Autodesk Inventor part; units mm, degrees
ref_plane "YZ Plane" through (0, 0, 0) normal (1, 0, 0) x (0, 1, 0)
ref_plane "XZ Plane" through (0, 0, 0) normal (0, 1, 0) x (-1, 0, 0)
ref_plane "XY Plane" through (0, 0, 0) normal (0, 0, 1) x (1, 0, 0)
sketch "Sketch1" plane through (0, 0, 0) normal (0, 1, 0) x (-1, 0, 0)
  line L0 (0, 0) -> (-76.5, 0)
  line L1 (-76.5, 0) -> (-76.5, 56.5)
  line L2 (-76.5, 56.5) -> (0, 56.5)
  line L3 (0, 56.5) -> (0, 0)
  dimension "d0" = 76.5
  dimension "d1" = 56.5
extrude "Extrusion1" add sketch "Sketch1" along normal blind 2
ref_plane "Work Plane1" through (0, 0, 28.25) normal (0, 0, 1) x (1, 0, 0)
ref_plane "Work Plane2" through (38.25, 0, 0) normal (-1, 0, 0) x (0, 0, 1)
sketch "Sketch2" plane through (0, 2, 0) normal (0, 1, 0) x (1, 0, 0)
  line L0 (38.25, -67.8) -> (38.25, 11.3) construction
  line L1 (91.8, -28.25) -> (-15.3, -28.25) construction
  line L2 (7.25, -7.25) -> (69.25, -7.25) construction
  line L3 (69.25, -7.25) -> (69.25, -49.25) construction
  line L4 (69.25, -49.25) -> (7.25, -49.25) construction
  line L5 (7.25, -49.25) -> (7.25, -7.25) construction
  circle A0 centre (7.25, -7.25) radius 1.75
  circle A1 centre (69.25, -7.25) radius 1.75
  point P0 (0, 0)
  dimension "d4" = 62
  dimension "d5" = 42
  dimension "d6" = 3.5
  dimension "d7" = 3.5
sketch "Sketch3" plane through (0, 2, 0) normal (0, 1, 0) x (1, 0, 0)
  line L0 (76.5, 0) -> (0, 0)
  line L1 (0, 0) -> (0, -56.5)
  line L2 (0, -56.5) -> (76.5, -56.5)
  line L3 (76.5, -56.5) -> (76.5, 0)
  line L4 (0, -56.5) -> (0, 0)
  line L5 (0, -17.5) -> (7.25, -17.5)
  line L6 (7.25, -17.5) -> (7.25, -49.5)
  line L7 (7.25, -49.5) -> (69.25, -49.5)
  line L8 (69.25, -49.5) -> (69.25, -17.5)
  line L9 (69.25, -17.5) -> (76.5, -17.5)
  line L10 (38.25, -67.8) -> (38.25, 11.3) construction
  dimension "d12" = 62
  dimension "d13" = 7
  dimension "d14" = 39
extrude "Extrusion3" cut sketch "Sketch3" against normal up to surface (2 mm away) contours L3 L2 L1 L5 L6 L7 L8 L9
extrude "Extrusion4" cut sketch "Sketch2" against normal up to surface (2 mm away)
sketch "Sketch4" plane through (0, 0, 0) normal (0, -1, 0) x (1, 0, 0)
  line L0 (7.25, 17.5) -> (0, 17.5)
  line L1 (7.25, 49.5) -> (7.25, 17.5)
  line L2 (69.25, 49.5) -> (7.25, 49.5)
  line L3 (69.25, 17.5) -> (69.25, 49.5)
  line L4 (76.5, 17.5) -> (69.25, 17.5)
  line L5 (0, 17.5) -> (0, 0)
  line L6 (76.5, 0) -> (76.5, 17.5)
  line L7 (9.25, 15.5) -> (9.25, 47.5)
  line L8 (9.25, 47.5) -> (67.25, 47.5)
  line L9 (67.25, 47.5) -> (67.25, 15.5)
  line L10 (67.25, 15.5) -> (74.5, 15.5)
  line L11 (74.5, 15.5) -> (74.5, 17.5)
  line L12 (69.25, 17.5) -> (76.5, 17.5)
  line L13 (9.25, 15.5) -> (2, 15.5)
  line L14 (2, 15.5) -> (2, 17.5)
  dimension "d20" = 2
  dimension "d21" = 2
  dimension "d22" = 2
  dimension "d25" = 2
  dimension "d26" = 2
  dimension "d27" = 2
extrude "Extrusion5" add sketch "Sketch4" along normal blind 4
sketch "Sketch5" plane through (69.25, 2, 49.5) normal (1, 0, 0) x (0, 0, -1)
  line L0 (32, 0) -> (32, -6) construction
  line L1 (0, 0) -> (32, 0) construction
  line L2 (0, 0) -> (0, -6) construction
  line L3 (32, -6) -> (0, -6) construction
  circle A0 centre (27.5, -2.75) radius 1.6
  point P0 (49.5, -2)
  dimension "d28" = 3.2
  dimension "d29" = 2.75
  dimension "d30" = 4.5
extrude "Extrusion6" cut sketch "Sketch5" against normal up to surface (2 mm away)
sketch "Sketch6" plane through (67.25, -4, 15.5) normal (-1, 0, 0) x (0, 0, 1)
  arc A0 (5.0867, 4) -> (7.9133, 4) centre (6.5, 3.25) ccw
  line L0 (0, 4) -> (5.0867, 4)
  line L1 (7.9133, 4) -> (32, 4)
  line L2 (9.5, 4) -> (3.5, 4)
  line L3 (3.5, 4) -> (3.5, 0)
  line L4 (3.5, 0) -> (9.5, 0)
  line L5 (9.5, 0) -> (9.5, 4)
  line L6 (6.5, 3.25) -> (6.5, 4) construction
  point P0 (-15.5, 4)
  dimension "d33" = 6
  dimension "d34" = 4
extrude "Extrusion7" add sketch "Sketch6" along normal blind 3.5
sketch "Sketch7" plane through (67.25, -0.75, 22) normal (1, 0, 0) x (0, 0, -1)
  circle A0 centre (0, 0) radius 1.6
  point P0 (22, 0.75)
extrude "Extrusion8" cut sketch "Sketch7" against normal up to surface (3.5 mm away)
sketch "Sketch8" plane through (0, -4, 0) normal (0, -1, 0) x (1, 0, 0)
  line L0 (7.25, 17.5) -> (2, 17.5)
  line L1 (2, 17.5) -> (2, 15.5)
  line L2 (2, 15.5) -> (9.25, 15.5)
  line L3 (9.25, 15.5) -> (9.25, 47.5)
  line L4 (9.25, 47.5) -> (67.25, 47.5)
  line L5 (67.25, 47.5) -> (67.25, 25)
  line L6 (67.25, 15.5) -> (74.5, 15.5)
  line L7 (74.5, 15.5) -> (74.5, 17.5)
  line L8 (74.5, 17.5) -> (69.25, 17.5)
  line L9 (69.25, 17.5) -> (69.25, 49.5)
  line L10 (69.25, 49.5) -> (7.25, 49.5)
  line L11 (7.25, 49.5) -> (7.25, 17.5)
  line L12 (73.5, 17.5) -> (73.5, 53.5)
  line L13 (73.5, 53.5) -> (3, 53.5)
  line L14 (3, 53.5) -> (3, 17.5)
  line L15 (74.5, 17.5) -> (69.25, 17.5)
  line L16 (7.25, 17.5) -> (2, 17.5)
  line L17 (67.25, 25) -> (63.75, 25) construction
  line L18 (63.75, 19) -> (63.75, 25) construction
  line L19 (67.25, 19) -> (63.75, 19) construction
  line L20 (67.25, 19) -> (67.25, 15.5)
  line L21 (67.25, 25) -> (67.25, 19)
  point P0 (0, 0)
  dimension "d39" = 53.5
  dimension "d65" = 1
  dimension "d66" = 1
extrude "Extrusion9" add sketch "Sketch8" along normal blind 2
fillet "Fillet1" radius 4 4 edges at (0, 1, 0) (76.5, 1, 0) (3, -5, 53.5) (73.5, -5, 53.5)
fillet "Fillet2" radius 4 4 edges at (7.25, -1, 49.5) (69.25, -1, 49.5) (9.25, -3, 47.5) (67.25, -3, 47.5)
sketch "Sketch9" plane through (0, 0, 0) normal (0, -1, 0) x (1, 0, 0)
  circle A0 centre (69.25, 7.25) radius 1.75
  circle A1 centre (7.25, 7.25) radius 1.75
  line L0 (72.25, 10.25) -> (66.25, 10.25)
  line L1 (66.25, 10.25) -> (66.25, 4.25)
  line L2 (66.25, 4.25) -> (72.25, 4.25)
  line L3 (72.25, 4.25) -> (72.25, 10.25)
  line L4 (72.25, 10.25) -> (66.25, 4.25) construction
  line L5 (66.25, 10.25) -> (72.25, 4.25) construction
  line L6 (10.25, 10.25) -> (4.25, 10.25)
  line L7 (4.25, 10.25) -> (4.25, 4.25)
  line L8 (4.25, 4.25) -> (10.25, 4.25)
  line L9 (10.25, 4.25) -> (10.25, 10.25)
  line L10 (10.25, 10.25) -> (4.25, 4.25) construction
  line L11 (4.25, 10.25) -> (10.25, 4.25) construction
  point P0 (0, 0)
  dimension "d44" = 6
  dimension "d45" = 6
  dimension "d46" = 6
  dimension "d47" = 6
extrude "Extrusion10" add sketch "Sketch9" along normal blind 5
sketch "Sketch10" plane through (0, 2, 0) normal (0, 1, 0) x (1, 0, 0)
  circle A0 centre (69.25, -7.25) radius 1.75
  circle A1 centre (7.25, -7.25) radius 1.75
  point P0 (0, 0)
extrude "Extrusion11" add sketch "Sketch10" against normal blind 1
sketch "Sketch11" plane through (0, -4, 0) normal (0, 1, 0) x (1, 0, 0)
  circle A0 centre (7.25, -7.25) radius 1.75 construction
  circle A1 centre (69.25, -7.25) radius 1.75 construction
  circle A2 centre (69.25, -7.25) radius 1.75 construction
  line L0 (7.25, -7.25) -> (69.25, -7.25) construction
  line L1 (69.25, -7.25) -> (69.25, -49.25) construction
  line L2 (69.25, -49.25) -> (7.25, -49.25) construction
  line L3 (7.25, -49.25) -> (7.25, -7.25) construction
  circle A3 centre (7.25, -49.25) radius 1.6
  circle A4 centre (69.25, -49.25) radius 1.6
  point P0 (0, 0)
  dimension "d52" = 3.2
  dimension "d53" = 3.2
  dimension "d54" = 42
extrude "Extrusion12" cut sketch "Sketch11" against normal up to surface (2 mm away)
sketch "Sketch14" plane through (0, -6, 0) normal (0, -1, 0) x (1, 0, 0)
  arc A0 (73.5, 49.5) -> (69.5, 53.5) centre (69.5, 49.5) ccw
  line L0 (73.5, 17.5) -> (73.5, 49.5)
  line L1 (69.5, 53.5) -> (7, 53.5)
  arc A1 (67.25, 43.5) -> (63.25, 47.5) centre (63.25, 43.5) ccw
  line L2 (67.25, 43.5) -> (67.25, 15.5)
  line L3 (13.25, 47.5) -> (63.25, 47.5)
  circle A2 centre (69.25, 49.25) radius 1.6
  line L4 (67.1791, 44.25) -> (73.5, 44.25)
  line L5 (63.25, 47.5) -> (13.25, 47.5)
  line L6 (64.25, 47.373) -> (64.25, 53.5)
  line L7 (69.5, 53.5) -> (7, 53.5)
  point P0 (0, 0)
  dimension "d67" = 5
  dimension "d68" = 5
extrude "Extrusion15" add sketch "Sketch14" along normal blind 1.5
sketch "Sketch15" plane through (0, -4, 0) normal (0, 1, 0) x (1, 0, 0)
  arc A0 (67.7939, -48.5868) -> (68.4944, -47.8397) centre (69.25, -49.25) ccw
  circle A1 centre (69.25, -49.25) radius 3
  point P0 (0, 0)
  dimension "d71" = 6
extrude "Extrusion16" cut sketch "Sketch15" along normal blind 4
mirror "Mirror2" about plane through (38.25, 0, 0) normal (-1, 0, 0) of "Extrusion16", "Extrusion15"
fillet "Fillet3" radius 2 8 edges at (7.25, 0, 10.25) (4.25, 0, 7.25) (7.25, 0, 4.25) (10.25, 0, 7.25) (69.25, 0, 4.25) (66.25, 0, 7.25) (72.25, 0, 7.25) (69.25, 0, 10.25)
mirror "Mirror4" about plane through (38.25, 0, 0) normal (-1, 0, 0) of "Extrusion6", "Extrusion7", "Extrusion8"
chamfer "Chamfer1" distance 3 angle 45 4 edges at (11, 0, 19) (11, 0, 25) (65.5, 0, 25) (65.5, 0, 19)
sketch "Sketch16" plane through (0, -4, 0) normal (0, 1, 0) x (1, 0, 0)
  circle A0 centre (7.25, -49.25) radius 1.6
  circle A1 centre (69.25, -49.25) radius 1.6
  point P0 (0, 0)
extrude "Extrusion17" [suppressed]
equation "\"d7\" = d6"
equation "\"d21\" = d20"
equation "\"d22\" = d21"
equation "\"d26\" = d25"
equation "\"d45\" = d44"
equation "\"d46\" = d45"
equation "\"d47\" = d45"
equation "\"d68\" = d67"
properties part number "case_back"
For this review, take the finished solid that the model builds, in its own axes (mm). A direction names the side the tool comes from. Give positions to 0.01 mm unless a question says otherwise; leave off trailing zeros. Order: outer loops, then holes, each group sorted by start corner. A loop starts at its lowest first (then second) coordinate and runs counter-clockwise, first axis right, second up.
1) Insertion check: pin 1 (0.7 mm diameter, centred on y = 0.5, z = 21.5, fed in from +X); pin 2 (1.8 mm diameter, centred on x = 70, z = 7, fed in from -Y); pin 3 (1.8 mm diameter, centred on y = -6, z = 37.5, fed in from +X). Each pin has a flat end and moves straight along its axis. Give the tip position at first contact, or say it passes through.
2) Take a section at B-B (x = 16.5). Give the boundary of the cut face in (y, z).
3) For faces 5 (the face through (64.25, -7, 50)), 6 (the face through (68, 0, 48)), 7 (the face through (68, -5, 9)), list the 3-axis set-ups (+Z, -Z, +X, -X, +Y, -Y) from which the entire face can be reached by the end or side of a thin tool; tool diameter is ignored.
4) Take a section at C-C (z = 39). Give the boundary of the cut face in (x, y), then the cut area to 3 significant figures.
5) The part is to be moulded in two halves that separate along X. For faces 1 (the face through (7, 1, 7)), 2 (the face through (10.391, -3.698, 46.297)), 3 (the face through (73.5, -5, 33)), 4 (the face through (9, -5, 6)), say which applies: released by +X, released by -X, zero draft, split by the parting line, or undercut.
6) Wall thickness on line 1 (Z direction, x = 69.25, y = -4.85); line 2 (X direction, y = -3.25, z = 20.5); line 3 (Z direction, x = 7.25, y = -6.15): over which ranges is each line inside the solid? List them lowest first.
7) Take a section at A-A (z = 22). Give the boundary of the cut face in (x, y).
Derived:
1. pin 1: stops at x = 69.25
1. pin 2: stops at y = 1
1. pin 3: stops at x = 73.5
2. outline: (-6, 47.5) - (0, 47.5) - (0, 0) - (2, 0) - (2, 49.5) - (-4, 49.5) - (-4, 53.5) - (-6, 53.5) - close
3. face 5: +Z, -Z, -Y
3. face 6: +Z, +X
3. face 7: -Z, +X, -X, -Y
4. outline: (3, -6) - (9.25, -6) - (9.25, 0) - (67.25, 0) - (67.25, -6) - (73.5, -6) - (73.5, -4) - (69.25, -4) - (69.25, 2) - (7.25, 2) - (7.25, -4) - (3, -4) - close
4. area: 165 mm2
5. face 1: undercut
5. face 2: undercut
5. face 3: released by +X
5. face 4: zero draft
6. line 1: z = 4.25 to 5.5, 9 to 10.25, 15.5 to 47.65, 50.85 to 53.5
6. line 2: x = 7.25 to 12.75, 63.75 to 69.25
6. line 3: z = 44.25 to 47.65, 50.85 to 53.5
7. outline: (3, -6) - (9.25, -6) - (9.25, -4) - (12.75, -4) - (12.75, -2.35) - (7.25, -2.35) - (7.25, -4) - (3, -4) - close; (7.25, 0.85) - (12.75, 0.85) - (12.75, 0) - (63.75, 0) - (63.75, 0.85) - (69.25, 0.85) - (69.25, 2) - (7.25, 2) - close; (63.75, -4) - (67.25, -4) - (67.25, -6) - (73.5, -6) - (73.5, -4) - (69.25, -4) - (69.25, -2.35) - (63.75, -2.35) - close
